Build history of the part. All positions in model axes, mm. A direction names the side the tool comes from. Give positions to 0.01 mm unless a question says otherwise; leave off trailing zeros. Write each loop counter-clockwise with the first axis right and the second up, starting at its lowest first coordinate (ties: lowest second). Pieces come first, ordered by that corner, then holes.
from build123d import *

# Parameters (mm, degrees)
SKETCH4_R               = 12.5
BOSS_EXTRUDE1_DEPTH     = 7
CUT_EXTRUDE1_DEPTH      = 32.336879232
CUT_EXTRUDE1_DEPTH_BACK = 32.336879232
SKETCH3_R               = 1.6
CUT_EXTRUDE2_DEPTH      = 33.031234756
CUT_EXTRUDE2_DEPTH_BACK = 33.031234756
SKETCH5_R               = 1.65
CUT_EXTRUDE3_DEPTH      = 2.7
CUT_EXTRUDE4_DEPTH      = 2.7


with BuildPart() as part:
    # Sketch2 → Revolve1 (revolve)
    with BuildSketch(Plane(origin=(0, 0, 0), x_dir=(1, 0, 0), z_dir=(0, 1, 0)), mode=Mode.PRIVATE) as revolve1_sk:
        Polygon((0, 5), (0, -5), (21, -5), (20, 0), (21, 5), align=None)
    revolve(revolve1_sk.sketch.rotate(Axis((0, 0, -5), (0, 0, 1)), 180), axis=Axis((0, 0, -5), (0, 0, 1)))

    # Sketch4 → Boss-Extrude1 (add)
    with BuildSketch(Plane(origin=(0, 0, -5), x_dir=(-1, 0, 0), z_dir=(0, 0, -1))):
        with Locations(Location((0, 0, 0), (0, 0, 180))):
            Circle(SKETCH4_R)
    extrude(amount=BOSS_EXTRUDE1_DEPTH)

    # Sketch3 → Cut-Extrude1 (cut, two sides: drawn at the far end of the back side and taken through both)
    with BuildSketch(Plane(origin=(0, 0, -5), x_dir=(-1, 0, 0), z_dir=(0, 0, -1)).offset(-CUT_EXTRUDE1_DEPTH_BACK)):
        Circle(SKETCH3_R)
    extrude(amount=CUT_EXTRUDE1_DEPTH + CUT_EXTRUDE1_DEPTH_BACK, mode=Mode.SUBTRACT)

    # Sketch5 → Cut-Extrude2 (cut, two sides: drawn at the far end of the back side and taken through both)
    with BuildSketch(Plane(origin=(0, 0, 0), x_dir=(0, 0, -1), z_dir=(1, 0, 0)).offset(-CUT_EXTRUDE2_DEPTH_BACK)):
        with Locations((8.5, 0)):
            Circle(SKETCH5_R)
    extrude(amount=CUT_EXTRUDE2_DEPTH + CUT_EXTRUDE2_DEPTH_BACK, mode=Mode.SUBTRACT)

    # Sketch6 → Cut-Extrude3 (cut)
    with BuildSketch(Plane(origin=(-3.2, 0, 0), x_dir=(0, 0, -1), z_dir=(1, 0, 0))):
        Polygon((10.145448267, 2.85), (12, 2.85), (12, -2.85), (10.145448267, -2.85), (6.854551733, -2.85), (5.209103466, 0), (6.854551733, 2.85), align=None)
    extrude(amount=-CUT_EXTRUDE3_DEPTH, mode=Mode.SUBTRACT)

    # Sketch7 → Cut-Extrude4 (cut)
    with BuildSketch(Plane(origin=(3.2, 0, 0), x_dir=(0, 0, -1), z_dir=(1, 0, 0))):
        Polygon((12, 2.85), (10.145448267, 2.85), (6.854551733, 2.85), (5.209103466, 0), (6.854551733, -2.85), (10.145448267, -2.85), (12, -2.85), align=None)
    extrude(amount=CUT_EXTRUDE4_DEPTH, mode=Mode.SUBTRACT)


solid = part.part
(1) Drop flat-ended pins along their axis: pin 1 (3 mm diameter, centred on y = 0, z = -8.5, fed in from +X); pin 2 (8 mm diameter, centred on y = -2.5, z = -8.5, fed in from -X); pin 3 (4 mm diameter, centred on x = 16, y = -2, fed in from -Z); pin 4 (6 mm diameter, centred on y = -15.5, z = -0.5, fed in from +X). Give the stop position or say it passes through.
(2) 3-axis set-ups, long thin cutter, end or side, ignore diameter. For faces 4 (the face through (-1.48, -0.61, -10.77)), 5 (the face through (-4.53, -1.44, -6.04)): which of +Z, -Z, +X, -X, +Y, -Y reach the whole face in a straight line?
(3) Saw through at C-C, the plane z = -2.5. List the corners of the cut face in (x, y), plus the area to 3 significant figures.
(4) Saw through at A-A, the plane x = 0. List the corners of the cut face in (y, z).
(5) Probe line 1 (Z direction, x = -8, y = 0); line 2 (Y direction, x = 0, z = -9.7); line 3 (Z direction, x = 9.5, y = -1). List the from-to ranges inside material, lowest first.
(6) Saw through at B-B, the plane z = 1.25. List the corners of the cut face in (x, y).
(7) Mould opens along Y. For faces 1 (the face through (9.154, 1.115, -7.284)), 2 (the face through (4, 0, 5)), 3 (the face through (-19.123, -6.022, 0.243)) say: +Y half, -Y half, draft (parallel to the pull), parting line (faces both ways), or undercut.
Computed values:
1. pin 1: passes through
1. pin 2: stops at x = -20.99
1. pin 3: stops at z = -5
1. pin 4: stops at x = 15.86
2. face 4: +Z, -Z
2. face 5: -Z
3. outline: circle Ø41 at (0, 0); hole circle Ø3.2 at (0, 0)
3. area: 1,310 mm2
4. outline: (-21, -5) - (-12.5, -5) - (-12.5, -12) - (-1.6, -12) - (-1.6, -8.9) arc R1.65 cw to (-1.6, -8.1) - (-1.6, 5) - (-21, 5) - (-20, 0) - close; (1.6, -12) - (12.5, -12) - (12.5, -5) - (21, -5) - (20, 0) - (21, 5) - (1.6, 5) - (1.6, -8.1) arc R1.65 cw to (1.6, -8.9) - close
5. line 1: z = -12 to -10.15, -6.85 to 5
5. line 2: y = -12.5 to -1.6, 1.6 to 12.5
5. line 3: z = -12 to -9.81, -7.19 to 5
6. outline: circle Ø40.5 at (0, 0); hole circle Ø3.2 at (0, 0)
7. face 1: undercut
7. face 2: draft
7. face 3: parting line
